Part model, mm, in its own coordinate system. A direction names the side the tool comes from. Coordinates: 2 decimals unless noted, no trailing zeros. Loops run counter-clockwise (first coordinate to the right, second up) from the corner with the lowest first, then second, coordinate; pieces in that order, holes last. Notation, with made-up numbers: (1, 2) - (14, 2) arc R21 ccw to (14, 15) - close; hole circle Ø2 at (25.5, -26). An arc over 180 degrees is marked (long way). Use a Markdown table: item, result. Add a question column.
1. Wall check: probe 1 along Y at (x, z) = (0, 1.6); probe 2 along Y at (x, z) = (1.75, 2.75); probe 3 along X at (y, z) = (1.75, 4.35). Give the ranges that are in metal, low to high. Write a range as [from, to].
2. Band-saw the part on B-B, the plane y = 12.7. Give the cut face in (x, z).
3. Band-saw the part on C-C, the plane z = 2.6. Give the cut face in (x, y).
4. Drop flat-ended pins along their axis: pin 1 (1.5 mm diameter, centred on y = 0.5, z = 3.5, fed in from +X); pin 2 (2.5 mm diameter, centred on y = 7, z = 3, fed in from +X); pin 3 (1.4 mm diameter, centred on y = 5, z = 3.5, fed in from -X). Give the stop position or say it passes through.
5. Band-saw the part on D-D, the plane y = 1.5. Give the cut face in (x, z), plus the area to 3 significant figures.
6. Band-saw the part on A-A, the plane x = 0. Give the cut face in (y, z).
7. Pull direction X, two halves, no side cores. Call faces 4 (the cylindrical face through (-0.44, 1.984, 2.379)), 5 (the flat face through (0, 7, 0)), 6 (the cylindrical face through (0.163, -5.077, 2.379)): pulls with the +X half, pulls with the -X half, needs draft (parallel to the pull), parting line crosses it, or undercut.
8. 3-axis set-ups, long thin cutter, end or side, ignore diameter. For faces 1 (the flat face through (3.81, 6, 2)), 2 (the flat face through (-3.81, 6, 2)), 3 (the cylindrical face through (-0.44, 14.684, 2.379)): which of +Z, -Z, +X, -X, +Y, -Y reach the whole face in a straight line?
Autodesk Inventor part; units mm, degrees
ref_plane "YZ Plane" through (0, 0, 0) normal (1, 0, 0) x (0, 1, 0)
ref_plane "XZ Plane" through (0, 0, 0) normal (0, 1, 0) x (-1, 0, 0)
ref_plane "XY Plane" through (0, 0, 0) normal (0, 0, 1) x (1, 0, 0)
sketch "Sketch1" plane through (0, 0, 0) normal (0, 0, 1) x (1, 0, 0)
  circle A0 centre (0, 0) radius 2.032
  arc A1 (-3.81, 3.3601) -> (3.81, 3.3601) centre (0, 0) ccw
  line L0 (-3.81, 3.3601) -> (-3.81, 9.3399)
  circle A2 centre (0, 12.7) radius 2.032
  arc A3 (3.81, 9.3399) -> (-3.81, 9.3399) centre (0, 12.7) ccw
  line L1 (3.81, 9.3399) -> (3.81, 3.3601)
  point P0 (-3.81, 6.35)
  dimension "d0" = 4.064
  dimension "d1" = 10.16
  dimension "d3" = 4.064
  dimension "d5" = 12.7
  dimension "d31" = 5.08
  dimension "d34" = 7.62
  dimension "d35" = 3.81
extrude "Extrusion1" add sketch "Sketch1" along normal blind 4.826
equation "\"d0\" = d3"
properties part number "Arm 1"
Geometry check:
| question | item | result |
|---|---|---|
| 1 | probe 1 | y = [-5.08, -2.03], [2.03, 10.67], [14.73, 17.78] |
| 1 | probe 2 | y = [-4.77, -1.03], [1.03, 11.67], [13.73, 17.47] |
| 1 | probe 3 | x = [-4.77, -1.03], [1.03, 4.77] |
| 2 | outline | (-5.08, 0) - (-2.03, 0) - (-2.03, 4.83) - (-5.08, 4.83) - close; (2.03, 0) - (5.08, 0) - (5.08, 4.83) - (2.03, 4.83) - close |
| 3 | outline | (-3.81, 3.36) arc R5.08 ccw (long way) to (3.81, 3.36) - (3.81, 9.34) arc R5.08 ccw (long way) to (-3.81, 9.34) - close; hole circle Ø4.06 at (0, 0); hole circle Ø4.06 at (0, 12.7) |
| 4 | pin 1 | stops at x = 5.08 |
| 4 | pin 2 | stops at x = 3.81 |
| 4 | pin 3 | stops at x = -3.81 |
| 5 | outline | (-4.85, 0) - (-1.37, 0) - (-1.37, 4.83) - (-4.85, 4.83) - close; (1.37, 0) - (4.85, 0) - (4.85, 4.83) - (1.37, 4.83) - close |
| 5 | area | 33.6 mm^2 |
| 6 | outline | (-5.08, 0) - (-2.03, 0) - (-2.03, 4.83) - (-5.08, 4.83) - close; (2.03, 0) - (10.67, 0) - (10.67, 4.83) - (2.03, 4.83) - close; (14.73, 0) - (17.78, 0) - (17.78, 4.83) - (14.73, 4.83) - close |
| 7 | face 4 | undercut |
| 7 | face 5 | needs draft |
| 7 | face 6 | parting line crosses it |
| 8 | face 1 | +Z, -Z, +X |
| 8 | face 2 | +Z, -Z, -X |
| 8 | face 3 | +Z, -Z |
